The listing builds one solid part. Answer for the finished solid, in the listing's coordinates (mm). A direction names the side the tool comes from. Round coordinates to 2 decimals unless told otherwise and drop trailing zeros. Loops run counter-clockwise (first coordinate to the right, second up) from the corner with the lowest first, then second, coordinate; pieces in that order, holes last. Notation, with made-up numbers: M -13,30 L 35,30 A21 ccw 35,44 Z; hole C -24,-20 d9. An arc over 180 degrees is marked long. Put each result on its own line as item: value. Start each with the question number.
(1) Straight lines are drawn through the part: line 1 (Y direction, x = 5, z = -5.25); line 2 (Y direction, x = 5, z = -2); line 3 (Y direction, x = 6.25, z = -10.5). For each, find the intervals that lie inside material, in ascending order.
(2) Which of the six approach directions +Z, -Z, +X, -X, +Y, -Y give full straight-line access (tool end or side, diameter ignored) to faces 1 (the face through (5, 5, -7.8)), 2 (the face through (5.85, 9.11, -4.06)), 3 (the face through (0, 21, -8)), 4 (the face through (5, 34, -5))?
(3) Section C-C, the plane x = 5 is taken. Determine the outline of the cut face in (y, z).
(4) Section D-D, the plane y = 5 is taken. Determine the outline of the cut face in (x, z), then the cut area to 3 significant figures.
(5) A flat-ended cylindrical pin translates along its axis: P1, Ø0.8, axis at x = 4.5, y = 29.5, coming from the +Z side. Find the tip coordinate at first contact, or state that the pin passes through.
(6) Section B-B, the plane z = -2.75 is taken. Determine the outline of the cut face in (x, y), then the cut area to 3 significant figures.
(7) Determine the mould class of faces 5 (the face through (5, 30, -8)), 6 (the face through (5, 21, 0)), 7 (the face through (10, 21, -8)) for opening direction X: released by +X, released by -X, zero draft, split by the parting line, or undercut.
(8) Section A-A, the plane y = 33 is taken. Determine the outline of the cut face in (x, z).
Autodesk Inventor part; units mm, degrees
ref_plane "YZ Plane" through (0, 0, 0) normal (1, 0, 0) x (0, 1, 0)
ref_plane "XZ Plane" through (0, 0, 0) normal (0, 1, 0) x (-1, 0, 0)
ref_plane "XY Plane" through (0, 0, 0) normal (0, 0, 1) x (1, 0, 0)
sketch "Эскиз1" plane through (0, 0, 0) normal (0, 1, 0) x (-1, 0, 0)
  line L0 (0, 0) -> (-10, 0)
  line L1 (-10, 0) -> (-10, -15.8)
  line L2 (-10, -15.8) -> (0, -15.8)
  line L3 (0, -15.8) -> (0, 0)
  dimension "d0" = 10
  dimension "d1" = 15.8
extrude "Выдавливание1" add sketch "Эскиз1" along normal blind 42
sketch "Эскиз2" plane through (10, 0, -15.8) normal (0, 0, -1) x (-1, 0, 0)
  line L0 (0, 0) -> (10, 0)
  line L1 (0, 42) -> (10, 42)
  point P0 (5, 5)
  point P1 (5, 37)
  point P2 (5, 0)
  dimension "d32" = 5
  dimension "d33" = 5
hole "Отверстие1" at (5, 5, -15.8) at (5, 37, -15.8) direction (0, 0, 1) diameter 2.8 depth 8
sketch "Эскиз3" plane through (10, 0, 0) normal (1, 0, 0) x (0, 0, -1)
  line L0 (0, 42) -> (15.8, 42)
  line L1 (0, 0) -> (15.8, 0)
  line L2 (15.8, 0) -> (15.8, 42)
  point P0 (9.8, 33)
  point P1 (9.8, 9)
  point P2 (7.9, 42)
  dimension "d34" = 9
  dimension "d35" = 9
  dimension "d37" = 6
hole "Отверстие2" at (10, 33, -9.8) at (10, 9, -9.8) direction (-1, 0, 0) diameter 2.8 end through all
sketch "Эскиз7" plane through (0, 42, 0) normal (0, 1, 0) x (1, 0, 0)
  line L0 (0, 0) -> (10, 0)
  point P0 (5, 5)
  point P1 (5, 0)
  dimension "d45" = 5
hole "Отверстие5" at (5, 42, -5) direction (0, -1, 0) diameter 2.8 depth 8
sketch "Эскиз9" plane through (0, 0, 0) normal (0, 0, 1) x (1, 0, 0)
  line L0 (0, 42) -> (10, 42)
  line L1 (0, 0) -> (10, 0)
  point P0 (5, 30)
  point P1 (5, 8)
  point P2 (5, 42)
  dimension "d53" = 12
  dimension "d54" = 8
hole "Отверстие6" at (5, 30, 0) at (5, 8, 0) direction (0, 0, -1) diameter 2.8 depth 8
properties part number "CupHolderBack"
Recorded:
1. line 1: y = 0 to 6.6, 9.4 to 28.6, 31.4 to 34
1. line 2: y = 0 to 6.6, 9.4 to 28.6, 31.4 to 42
1. line 3: y = 0 to 4.37, 5.63 to 7.79, 10.21 to 31.79, 34.21 to 36.37, 37.63 to 42
2. face 1: -Z
2. face 2: +Z
2. face 3: +Z, -Z, -X, +Y, -Y
2. face 4: +Y
3. outline: M 0,-15.8 L 3.6,-15.8 L 3.6,-7.8 L 6.4,-7.8 L 6.4,-15.8 L 35.6,-15.8 L 35.6,-7.8 L 38.4,-7.8 L 38.4,-15.8 L 42,-15.8 L 42,-6.4 L 34,-6.4 L 34,-3.6 L 42,-3.6 L 42,0 L 31.4,0 L 31.4,-8 L 28.6,-8 L 28.6,0 L 9.4,0 L 9.4,-8 L 6.6,-8 L 6.6,0 L 0,0 Z; hole C 9,-9.8 d2.8; hole C 33,-9.8 d2.8
4. outline: M 0,-15.8 L 3.6,-15.8 L 3.6,-7.8 L 6.4,-7.8 L 6.4,-15.8 L 10,-15.8 L 10,0 L 0,0 Z
4. area: 136 mm²
5. P1: stops at z = -8
6. outline: M 0,0 L 10,0 L 10,42 L 0,42 Z; hole C 5,8 d2.8; hole C 5,30 d2.8
6. area: 408 mm²
7. face 5: undercut
7. face 6: zero draft
7. face 7: released by +X
8. outline: M 0,-15.8 L 10,-15.8 L 10,-11.2 L 0,-11.2 Z; M 0,-8.4 L 10,-8.4 L 10,0 L 0,0 Z
